```python
from build123d import *

# Parameters (mm, degrees)
BOSS_EXTRUDE1_DEPTH = 5
SKETCH2_R           = 2.75
CUT_EXTRUDE1_DEPTH  = 53.376168941


with BuildPart() as part:
    # Sketch1 → Boss-Extrude1 (new body)
    with BuildSketch(Plane.XY):
        Polygon((22.999000463, 20.515274598), (32.999000463, 20.515274598), (32.999000463, 15.515274598), (37.999000463, 15.515274598), (37.999000463, 5.515274598), (42.999000463, 5.515274598), (42.999000463, -14.484725402), (37.999000463, -14.484725402), (37.999000463, -24.484725402), (32.999000463, -24.484725402), (32.999000463, -29.484725402), (22.999000463, -29.484725402), (22.999000463, -24.484725402), (17.999000463, -24.484725402), (17.999000463, -14.484725402), (12.999000463, -14.484725402), (12.999000463, 5.515274598), (17.999000463, 5.515274598), (17.999000463, 15.515274598), (22.999000463, 15.515274598), align=None)
    extrude(amount=BOSS_EXTRUDE1_DEPTH)

    # Sketch2 → Cut-Extrude1 (cut, through all)
    with BuildSketch(Plane.XY.offset(5)):
        with Locations((24.48386892, 10.515274598)):
            Circle(SKETCH2_R)
        with Locations((24.48386892, 0.515274598)):
            Circle(SKETCH2_R)
        with Locations((24.48386892, -9.484725402)):
            Circle(SKETCH2_R)
        with Locations((24.48386892, -19.484725402)):
            Circle(SKETCH2_R)
        with Locations(Location((31.514132006, -19.484725402, 0), (0, 0, 180))):
            Circle(SKETCH2_R)
        with Locations(Location((31.514132006, -9.484725402, 0), (0, 0, 180))):
            Circle(SKETCH2_R)
        with Locations(Location((31.514132006, 0.515274598, 0), (0, 0, 180))):
            Circle(SKETCH2_R)
        with Locations(Location((31.514132006, 10.515274598, 0), (0, 0, 180))):
            Circle(SKETCH2_R)
    extrude(amount=-CUT_EXTRUDE1_DEPTH, mode=Mode.SUBTRACT)


solid = part.part
```
The listing builds one solid part. Answer for the finished solid, in the listing's coordinates (mm). A direction names the side the tool comes from. Give positions to 0.01 mm unless a question says otherwise; leave off trailing zeros. Write each loop counter-clockwise with the first axis right and the second up, starting at its lowest first coordinate (ties: lowest second). Pieces come first, ordered by that corner, then holes. Notation, with made-up numbers: (-25.75, 74.5) -> (1.25, 74.5) arc R18 ccw to (1.25, 83.5) -> close; hole circle Ø9 at (2.25, 35). An arc over 180 degrees is marked (long way). Use one line per item in the form item = value.
1) Section A-A on x = 33.75 is taken. Write down the section's boundary in (y, z).
Result:
outline = (-24.48, 0) -> (-21.09, 0) -> (-21.09, 5) -> (-24.48, 5) -> close; (-17.88, 0) -> (-11.09, 0) -> (-11.09, 5) -> (-17.88, 5) -> close; (-7.88, 0) -> (-1.09, 0) -> (-1.09, 5) -> (-7.88, 5) -> close; (2.12, 0) -> (8.91, 0) -> (8.91, 5) -> (2.12, 5) -> close; (12.12, 0) -> (15.52, 0) -> (15.52, 5) -> (12.12, 5) -> close
2) Section B-B on y = 10 is taken. Write down the section's boundary in (x, z).
Result:
outline = (18, 0) -> (21.78, 0) -> (21.78, 5) -> (18, 5) -> close; (27.19, 0) -> (28.81, 0) -> (28.81, 5) -> (27.19, 5) -> close; (34.22, 0) -> (38, 0) -> (38, 5) -> (34.22, 5) -> close
3) Section C-C on z = 1.1 is taken. Count the separate pieces of the cut face and the enclosed holes in it, plus the area to 3 significant figures.
Result:
separate_pieces = 1
enclosed_holes = 8
area = 910 mm²
4) For a pull along Y with two mould halves and no side action, classify faces 5 (the flat face through (28, -4, 0)), 6 (the flat face through (40, 5.515, 2)), 7 (the cylindrical face through (21.737, 0.636, 2.535)) as +Y half, -Y half, draft (parallel to the pull), parting line (faces both ways), or undercut.
Result:
face_5 = draft
face_6 = +Y half
face_7 = undercut
5) A tool of negligible diameter and unlimited length cuts with its end or side. For faces 1 (the flat face through (20, 15.515, 2)), 2 (the flat face through (32.999, 18, 2)), 3 (the flat face through (17.999, -20, 2)), 4 (the flat face through (37.999, -19, 2)), from which of +Z, -Z, +X, -X, +Y, -Y can it reach the whole face along a straight path? Write none if from no direction.
Result:
face_1 = +Z, -Z, -X, +Y
face_2 = +Z, -Z, +X, +Y
face_3 = +Z, -Z, -X, -Y
face_4 = +Z, -Z, +X, -Y
6) Straight lines are drawn through the part: probe 1 along X at (y, z) = (-10, 1.7); probe 2 along X at (y, z) = (-10.5, 4.75); probe 3 along Y at (x, z) = (25.5, 2.55). For each, find the intervals that lie inside material, in ascending order.
Result:
probe_1 = 13 to 21.78, 27.19 to 28.81, 34.22 to 43
probe_2 = 13 to 21.93, 27.04 to 28.96, 34.07 to 43
probe_3 = -29.48 to -22.04, -16.93 to -12.04, -6.93 to -2.04, 3.07 to 7.96, 13.07 to 20.52
7) Each of these flat-tipped pins is pushed along its axis until it touches: P1, Ø1.5, axis at y = -28, z = 2, coming from the -X side; P2, Ø1.5, axis at x = 21.5, z = 2.5, coming from the -Y side; P3, Ø1.5, axis at x = 22.5, z = 1, coming from the +Y side; P4, Ø2.5, axis at y = -21, z = 3, coming from the +X side. Where does it stop, or does it pass through?
Result:
P1 = 23
P2 = -24.48
P3 = 20.52
P4 = 38
8) Section D-D on x = 39.25 is taken. Write down the section's boundary in (y, z).
Result:
outline = (-14.48, 0) -> (5.52, 0) -> (5.52, 5) -> (-14.48, 5) -> close
